The model under review builds one solid part; all positions refer to its coordinate system, in mm. A direction names the side the tool comes from. Round coordinates to 2 decimals unless told otherwise and drop trailing zeros. Order: outer loops, then holes, each group sorted by start corner. A loop starts at its lowest first (then second) coordinate and runs counter-clockwise, first axis right, second up. Notation, with made-up numbers: (10.5, -40) - (65.5, -40) arc R26 ccw to (65.5, -8) - close; hole circle Ø6 at (59, -20). An arc over 180 degrees is marked (long way). One line per question, with ' | ' between items. Start each with the question number.
Item 1: Add section C-C on y = -41. State the section outline as (x, z) points.
Item 2: Tool access review of faces 4 (the face through (28.575, 70, 13)), 5 (the face through (9.525, -70, 13)), 6 (the face through (19, 63.5, 15)), 7 (the face through (18.33, 73.07, 13.54)), 8 (the face through (19.5, -66.6, 15.7)): name each direction out of +Z, -Z, +X, -X, +Y, -Y from which nothing blocks a thin tool from reaching the whole face with its end or side.
Item 3: Add section B-B on x = 19.05. State how many separate pieces and enclosed holes the cut face has, and give its area (3 significant figures).
Item 4: Draft analysis for pull direction Z (two halves, no side actions). For faces 1 (the face through (19.259, -69.939, 28.573)), 2 (the face through (23, -69.85, 19)), 3 (the face through (19, -63.5, 15)), state which applies: +Z half, -Z half, draft (parallel to the pull), parting line (faces both ways), or undercut.
Item 5: For L1, parallel to Y at x = 19.05, z = 2.55 (3 decimals); L2, parallel to X at y = -88.9, z = 1.35 (3 decimals); L3, parallel to Y at x = 25, z = 19.75, list the stretches that pass through material, from the lowest coordinate up. Write a range as [from, to].
Item 6: Add section D-D on x = 31. State the section outline as (y, z) points, and give its area (3 significant figures).
Item 7: Add section A-A on z = 26.5. State the section outline as (x, y) points.
Item 8: Insertion check: pin 1 Ø5.5 at (x, z) = (22, 12.5) entering from -Y; pin 2 Ø6.5 at (y, z) = (-73, 15.5) entering from -X (3 decimals); pin 3 Ø10 at (y, z) = (-68, 15.5) entering from +X (3 decimals). Each pin has a flat end and moves straight along its axis. Give the tip position at first contact, or say it passes through.
from build123d import *

# Parameters (mm, degrees)
BOSS_EXTRUDE1_DEPTH                              = 6.35
SKETCH6_W                                        = 19.05
SKETCH6_H                                        = 12.7
BOSS_EXTRUDE4_DEPTH                              = 12.7
BOSS_EXTRUDE7_DEPTH                              = 12.7
CBORE_FOR_1_4_SOCKET_HEAD_CAP_SCREW1_D           = 6.7564
CBORE_FOR_1_4_SOCKET_HEAD_CAP_SCREW1_CBORE_D     = 11.1125
CBORE_FOR_1_4_SOCKET_HEAD_CAP_SCREW1_CBORE_DEPTH = 6.35


with BuildPart() as part:
    # Sketch1 → Boss-Extrude1 (new body)
    with BuildSketch(Plane.XY):
        with BuildLine():
            Line((0, 0), (0, 88.9))
            ThreePointArc((0, 88.9), (19.05, 107.95), (38.1, 88.9))
            Line((38.1, 88.9), (38.1, 0))
            Line((38.1, 0), (0, 0))
        make_face()
    extrude(amount=BOSS_EXTRUDE1_DEPTH)

    # Sketch5 → CSK for 5/16 Flat Head Machine Screw (100)1 (revolve, cut)
    with BuildSketch(Plane(origin=(19.05, 88.9, 6.35), x_dir=(0, -1, 0), z_dir=(1, 0, 0))):
        Polygon((0, 0), (0, 6.35), (4.36499, 6.35), (4.36499, 3.104257477), (8.0645, 0), align=None)
    revolve(axis=Axis((19.05, 88.9, 12.7), (0, 0, -1)), mode=Mode.SUBTRACT)

    # Sketch6 → Boss-Extrude4 (add)
    with BuildSketch(Plane.XY.offset(6.35)):
        with Locations((19.05, 69.85)):
            Rectangle(SKETCH6_W, SKETCH6_H)
    extrude(amount=BOSS_EXTRUDE4_DEPTH)

    # Sketch12 → Boss-Extrude7 (add)
    with BuildSketch(Plane(origin=(0, 76.2, 0), x_dir=(1, 0, 0), z_dir=(0, 1, 0))):
        with BuildLine():
            Line((9.525, -19.05), (28.575, -19.05))
            ThreePointArc((28.575, -19.05), (19.05, -28.575), (9.525, -19.05))
        make_face()
    extrude(amount=-BOSS_EXTRUDE7_DEPTH)

    # CBORE for 1/4 Socket Head Cap Screw1 (through all)
    with Locations(Plane(origin=(0, 76.2, 0), x_dir=(1, 0, 0), z_dir=(0, 1, 0))):
        with Locations((19.05, -19.05)):
            CounterBoreHole(CBORE_FOR_1_4_SOCKET_HEAD_CAP_SCREW1_D / 2, CBORE_FOR_1_4_SOCKET_HEAD_CAP_SCREW1_CBORE_D / 2, CBORE_FOR_1_4_SOCKET_HEAD_CAP_SCREW1_CBORE_DEPTH)

    # Mirror1: part across plane


with BuildPart() as part_1:
    add(part.part)
    add(part.part.mirror(Plane(origin=(38.1, 0, 6.35), x_dir=(0, 0, 1), z_dir=(0, 1, 0))))


solid = part_1.part
Determined:
1) outline: (0, 0) - (38.1, 0) - (38.1, 6.35) - (0, 6.35) - close
2) face 4: +Z, +X, +Y, -Y | face 5: +Z, -X, +Y, -Y | face 6: +Z, +X, -X | face 7: +Y | face 8: +Y, -Y
3) separate pieces: 5 | enclosed holes: 0 | area: 1,570 mm2
4) face 1: +Z half | face 2: undercut | face 3: draft
5) L1: [-107.95, -93.265], [-84.535, 84.535], [93.265, 107.95] | L2: [0, 14.685], [23.415, 38.1] | L3: [-76.2, -63.5], [63.5, 76.2]
6) outline: (-103.74, 0) - (103.74, 0) - (103.74, 6.35) - (-103.74, 6.35) - close | area: 1,320 mm2
7) outline: (13.12, -76.2) - (24.98, -76.2) - (24.98, -63.5) - (13.12, -63.5) - close; (13.12, 63.5) - (24.98, 63.5) - (24.98, 76.2) - (13.12, 76.2) - close
8) pin 1: y = -76.2 | pin 2: x = 9.525 | pin 3: x = 28.575
